Can you work these out from the model? Positions are in its coordinate system, mm. Face numbers are marked on the shaded views. A direction names the side the tool comes from. Give positions to 0.01 mm unless a question says otherwise; leave off trailing zeros. Loops run counter-clockwise (first coordinate to the right, second up) from the corner with the lowest first, then second, coordinate; pieces in that order, holes last. Notation, with made-up numbers: M 81.25,61.5 L 130.25,61.5 A22 ccw 130.25,100.5 Z; hole C -37.5,54 d1. An arc over 180 degrees is marked long. Use CSV: the item, a comma, the result in double quotes.
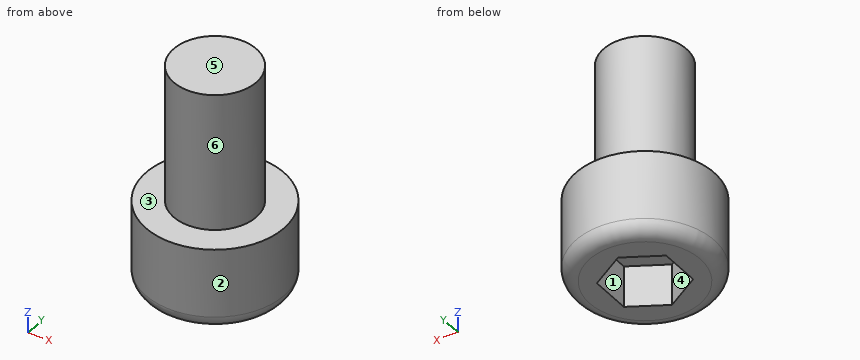
from build123d import *

# Parameters (mm, degrees)
SKETCH_1_R          = 5
EXTRUDE_1_DEPTH     = 6
SKETCH_2_R          = 3
EXTRUDE_2_DEPTH     = 10
CUT_EXTRUDE_1_DEPTH = 3
FILLET_1_R          = 1


with BuildPart() as part:
    # ｽｹｯﾁ1 → ﾎﾞｽ - 押し出し1 (new body)
    with BuildSketch(Plane.XY):
        Circle(SKETCH_1_R)
    extrude(amount=EXTRUDE_1_DEPTH)

    # ｽｹｯﾁ2 → ﾎﾞｽ - 押し出し2 (add)
    with BuildSketch(Plane.XY.offset(6)):
        Circle(SKETCH_2_R)
    extrude(amount=EXTRUDE_2_DEPTH)

    # ｽｹｯﾁ3 → ｶｯﾄ - 押し出し1 (cut)
    with BuildSketch(Plane(origin=(0, 0, 0), x_dir=(-1, 0, 0), z_dir=(0, 0, -1))):
        Polygon((-2.5, -1.443375673), (0, -2.886751346), (2.5, -1.443375673), (2.5, 1.443375673), (0, 2.886751346), (-2.5, 1.443375673), align=None)
    extrude(amount=-CUT_EXTRUDE_1_DEPTH, mode=Mode.SUBTRACT)

    # ﾌｨﾚｯﾄ1
    fillet_1_edges = [part.edges().sort_by_distance(p)[0] for p in [
        (-5, 0, 0),
    ]]
    fillet(fillet_1_edges, radius=FILLET_1_R)


solid = part.part
Q1. If we mould it in two halves opening along X, with no side actions, what happens to the marked faces 1, 2 and 3? For each: released by +X, released by -X, zero draft, split by the parting line, or undercut.
Model answer:
face 1,"undercut"
face 2,"split by the parting line"
face 3,"zero draft"
Q2. I want a section at B-B, the plane y = 0. Please give me the cut outline in (x, z).
Model answer:
outline,"M -5,1 A1 ccw -4,0 L -2.5,0 L -2.5,3 L 2.5,3 L 2.5,0 L 4,0 A1 ccw 5,1 L 5,6 L 3,6 L 3,16 L -3,16 L -3,6 L -5,6 Z"
Q3. I want a section at A-A, the plane z = 2.25. Please give me the cut outline in (x, y).
Model answer:
outline,"C 0,0 d10; hole M -2.5,-1.44 L 0,-2.89 L 2.5,-1.44 L 2.5,1.44 L 0,2.89 L -2.5,1.44 Z"
Q4. I want a section at C-C, the plane z = 4.5. Please give me the cut outline in (x, y), then the cut area to 3 significant figures.
Model answer:
outline,"C 0,0 d10"
area,"78.5 mm2"
Q5. Please list where these lines run through material, in increasing order: L1, parallel to Y at x = 0, z = 15; L2, parallel to Z at x = 0.75, y = -2.25; L3, parallel to Y at x = 1.25, z = 1. Write a range as from..to.
Model answer:
L1,"-3..3"
L2,"3..16"
L3,"-4.84..-2.17, 2.17..4.84"
Q6. I want a section at D-D, the plane z = 15. Please give me the cut outline in (x, y).
Model answer:
outline,"C 0,0 d6"
Q7. I'm going to push flat-ended pins straight in: P1, Ø4, axis at y = -0.5, z = 8.5, coming from the -X side; P2, Ø2, axis at x = 1.5, z = 13.5, coming from the -Y side; P3, Ø1, axis at y = -1.5, z = 5, coming from the +X side. Where does each tip first touch, or does it pass through?
Model answer:
P1,"x = -3"
P2,"y = -2.96"
P3,"x = 4.9"
Q8. For the marked faces 4, 5 and 6, which set-ups out of +Z, -Z, +X, -X, +Y, -Y let a thin tool reach every point of the face, with its end or its side?
Model answer:
face 4,"-Z"
face 5,"+Z, +X, -X, +Y, -Y"
face 6,"+Z"
